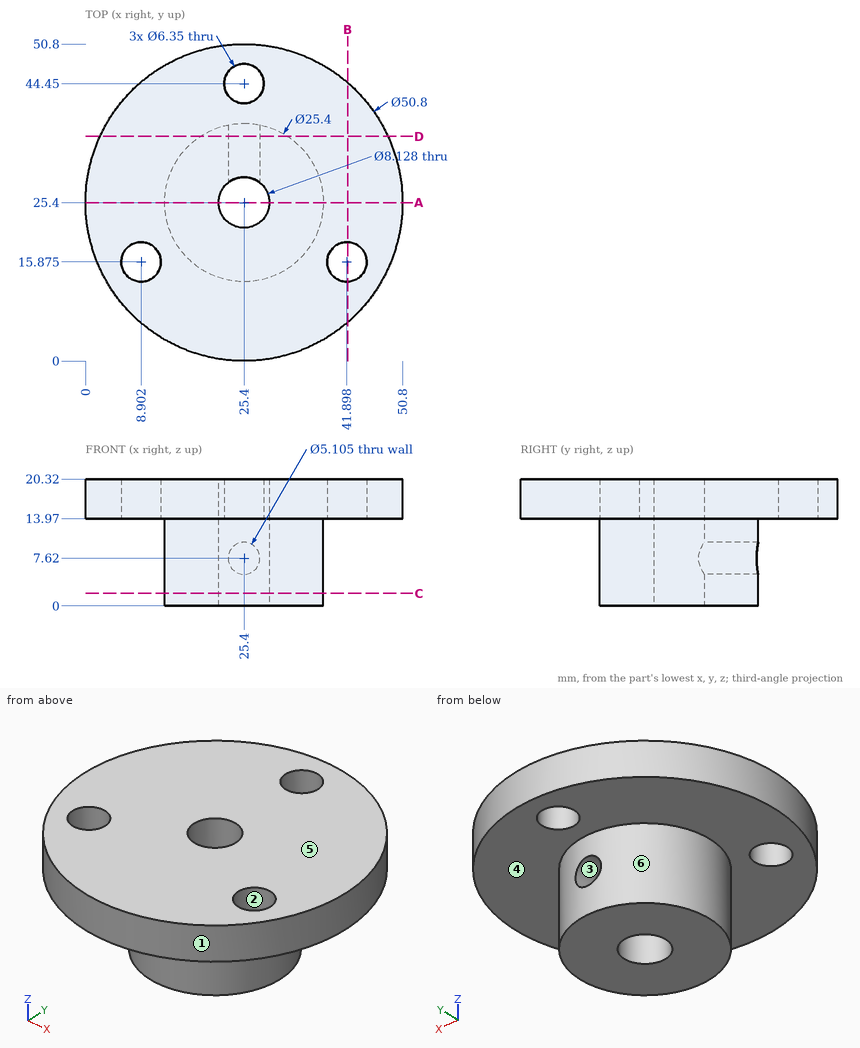
Geometry: see drawing. Coordinates: mm, zero at the bounding-box minimum. A direction names the side the tool comes from. Coordinates: 2 decimals unless noted, no trailing zeros. Order: outer loops, then holes, each group sorted by start corner. A loop starts at its lowest first (then second) coordinate and runs counter-clockwise, first axis right, second up. Notation, with made-up numbers: (85, 75) - (137, 75) arc R23 cw to (137, 111) - close; hole circle Ø2 at (-26, 14.25). An arc over 180 degrees is marked (long way). Return JSON: item names as keys, results as strings.
Q1. Access query for the marked faces 5 and 6. Directions: +Z, -Z, +X, -X, +Y, -Y. A direction counts if a zero-diameter tool reaches every point of the face in a straight line with its end or side. Return the directions, or none.
The answers:
{"face 5": "+Z, +X, -X, +Y, -Y", "face 6": "-Z"}
Q2. Cut plane A-A (y = 25.4). Return loops of the section in (x, z), then the cut area to 3 significant figures.
The answers:
{"outline": "(0, 13.97) - (12.7, 13.97) - (12.7, 0) - (21.34, 0) - (21.34, 20.32) - (0, 20.32) - close; (29.46, 0) - (38.1, 0) - (38.1, 13.97) - (50.8, 13.97) - (50.8, 20.32) - (29.46, 20.32) - close", "area": "512 mm2"}
Q3. Cut plane D-D (y = 36). Return loops of the section in (x, z) (1 decimal).
The answers:
{"outline": "(2.3, 14) - (18.4, 14) - (18.4, 0) - (32.4, 0) - (32.4, 14) - (48.5, 14) - (48.5, 20.3) - (2.3, 20.3) - close; hole circle Ø5.1 at (25.4, 7.6)"}
Q4. Cut plane B-B (x = 42). Return loops of the section in (y, z) (1 decimal), then the cut area to 3 significant figures.
The answers:
{"outline": "(6.2, 14) - (12.7, 14) - (12.7, 20.3) - (6.2, 20.3) - close; (19, 14) - (44.6, 14) - (44.6, 20.3) - (19, 20.3) - close", "area": "204 mm2"}
Q5. Cut plane C-C (z = 2). Return loops of the section in (x, y).
The answers:
{"outline": "circle Ø25.4 at (25.4, 25.4); hole circle Ø8.13 at (25.4, 25.4)"}
Q6. First-contact query: pin 1 (1.5 mm diameter, centred on x = 29.5, z = 17.5, fed in from -Y); pin 2 (10 mm diameter, centred on x = 6, z = 16.5, fed in from +Y); pin 3 (1.5 mm diameter, centred on y = 11.5, z = 10, fed in from -X); pin 4 (10 mm diameter, centred on x = 21, z = 11.5, fed in from +Y). Flat tips, straight axial feed; report the tip coordinate or a pass-through.
The answers:
{"pin 1": "stops at y = 0.22", "pin 2": "stops at y = 46.32", "pin 3": "passes through", "pin 4": "stops at y = 50.8"}
Q7. Ray query, probe 1 along Y at (x, z) = (25.5, 13); probe 2 along Y at (x, z) = (26, 19); probe 3 along Z at (x, y) = (25.4, 36.25). Return the intervals inside material, ascending.
The answers:
{"probe 1": "y = 12.7 to 21.34, 29.46 to 38.1", "probe 2": "y = 0.01 to 21.38, 29.42 to 41.33, 47.57 to 50.79", "probe 3": "z = 0 to 5.07, 10.17 to 20.32"}
Q8. Draft query along X for the marked faces 1, 2, 3 and 4. Return one class per face: +X half, -X half, draft (parallel to the pull), parting line (faces both ways), or undercut.
The answers:
{"face 1": "parting line", "face 2": "undercut", "face 3": "undercut", "face 4": "draft"}
